from build123d import *

# Parameters (mm, degrees)
F2_W     = 6.671602
F2_H     = 2
F2_W_2   = 14.827402
F3_DEPTH = 12.5


with BuildPart() as f1:
    # F0 (on Front) → F1 (revolve)
    with BuildSketch(Plane.XZ):
        Polygon((-7.055335, 2.8), (-7.055335, 0), (18.944665, 0), (18.944665, 2.8), (18.444665, 3.3), (16.444665, 3.3), (16.444665, 2.8), (-4.555335, 2.8), (-4.555335, 3.3), (-6.555335, 3.3), align=None)
    revolve(axis=Axis((5.944665, 0, 0), (1, 0, 0)))

    # F2 (on Top) → F3 (cut, symmetric)
    with BuildSketch(Plane.XY):
        with Locations((-5.391136, 0)):
            Rectangle(F2_W, F2_H)
        with Locations((21.358366, 0)):
            Rectangle(F2_W_2, F2_H)
    extrude(amount=F3_DEPTH, both=True, mode=Mode.SUBTRACT)


solid = f1.part
The listing builds one solid part. Answer for the finished solid, in the listing's coordinates (mm). A direction names the side the tool comes from. Round coordinates to 2 decimals unless told otherwise and drop trailing zeros. Order: outer loops, then holes, each group sorted by start corner. A loop starts at its lowest first (then second) coordinate and runs counter-clockwise, first axis right, second up. Notation, with made-up numbers: (21, 57.25) -> (28, 57.25) arc R28 cw to (28, 78.25) -> close; hole circle Ø2 at (16, -33.5). An arc over 180 degrees is marked (long way). One line per item, written item: value.
Item 1: Find section B-B, the plane y = 0. Give the vertices of the cut face in (x, z).
Taken from the geometry:
outline: (-2.06, -2.8) -> (13.94, -2.8) -> (13.94, 2.8) -> (-2.06, 2.8) -> close
Item 2: Find section A-A, the plane z = 0. Give the vertices of the cut face in (x, y), then the cut area to 3 significant figures.
Taken from the geometry:
outline: (-7.06, -2.8) -> (-6.56, -3.3) -> (-4.56, -3.3) -> (-4.56, -2.8) -> (16.44, -2.8) -> (16.44, -3.3) -> (18.44, -3.3) -> (18.94, -2.8) -> (18.94, -1) -> (13.94, -1) -> (13.94, 1) -> (18.94, 1) -> (18.94, 2.8) -> (18.44, 3.3) -> (16.44, 3.3) -> (16.44, 2.8) -> (-4.56, 2.8) -> (-4.56, 3.3) -> (-6.56, 3.3) -> (-7.06, 2.8) -> (-7.06, 1) -> (-2.06, 1) -> (-2.06, -1) -> (-7.06, -1) -> close
area: 130 mm2
Item 3: Straight lines are drawn through the part: L1, parallel to Y at x = -2.25, z = 1; L2, parallel to Y at x = -4, z = 0; L3, parallel to Y at x = 2.5, z = 1.25. For each, find the intervals that lie inside material, in ascending order.
Taken from the geometry:
L1: y = -2.62 to -1, 1 to 2.62
L2: y = -2.8 to -1, 1 to 2.8
L3: y = -2.51 to 2.51
Item 4: For faces 5 (the flat face through (-4.555, -3, 0)), 6 (the cylindrical face through (5.798, 2.733, -0.607)), 7 (the flat face through (16, 1, 0)), determine the directions among +Z, -Z, +X, -X, +Y, -Y from which every point of the face is accessible in a straight line to the end or side of a thin tool.
Taken from the geometry:
face 5: -Y
face 6: none
face 7: +Z, -Z, +X
Item 5: For a pull along X with two mould halves and no side action, classify faces 1 (the flat face through (-4.555, 3, 0)), 2 (the flat face through (16.445, 3, 0)), 3 (the flat face through (-2.055, 0, 0)), 4 (the flat face through (18.945, -2, 0)) as released by +X, released by -X, zero draft, split by the parting line, or undercut.
Taken from the geometry:
face 1: undercut
face 2: undercut
face 3: released by -X
face 4: released by +X
Item 6: Given P1, Ø3, axis at x = 2, z = 1.5, coming from the -Y side; P2, Ø1.5, axis at x = 17, z = -1.5, coming from the +Y side; P3, Ø1.5, axis at y = 0, z = -1.5, coming from the -X side, each flat-ended and moving along its own axis, determine where each tip first touches the part or whether it passes through.
Taken from the geometry:
P1: stops at y = -2.8
P2: stops at y = 3.21
P3: stops at x = -2.06
Item 7: Find section C-C, the plane x = 5.5. Give the vertices of the cut face in (y, z).
Taken from the geometry:
outline: circle Ø5.6 at (0, 0)
